```python
from build123d import *

# Parameters (mm, degrees)
F0_R          = 2
F1_DEPTH      = 20
F3_DEPTH      = 3
F3_DEPTH_BACK = 3
F6_DEPTH      = 1
F9_DEPTH      = 1
F10_DEPTH     = 20


with BuildPart() as f1:
    # F0 (on Front) → F1 (new body)
    with BuildSketch(Plane.XZ):
        with BuildLine():
            ThreePointArc((-3, 0), (0, -3), (3, 0))
            ThreePointArc((3, 0), (2.1213203436, 2.1213203436), (0, 3))
            ThreePointArc((0, 3), (-2.1213203436, 2.1213203436), (-3, 0))
        make_face()
        Circle(F0_R, mode=Mode.SUBTRACT)
    extrude(amount=F1_DEPTH)

    # F2 (on Right) → F3 (join, two sides)
    with BuildSketch(Plane.YZ) as f3_sk:
        Polygon((-5.2886751346, -7.6961524227), (-2, -2), (-3.1547005384, -2), (-6.1547005384, -7.1961524227), align=None)
        Polygon((-9.1547005384, -7.1961524227), (-6.1547005384, -2), (-7.3094010768, -2), (-10.0207259422, -6.6961524227), align=None)
    extrude(amount=F3_DEPTH)
    extrude(f3_sk.sketch, amount=-F3_DEPTH_BACK)

    # F5 (on offset) → F6 (join)
    with BuildSketch(Plane(origin=(0, -0.6339745962, 0.3660254038), x_dir=(-1, 0, 0), z_dir=(0, 0.8660254038, -0.5))):
        Polygon((3, -4), (3, 0), (1.5, -4), align=None)
        Polygon((-1.5, -4), (-3, 0), (-3, -4), align=None)
    extrude(amount=-F6_DEPTH)

    # F8 (on offset) → F9 (join)
    with BuildSketch(Plane(origin=(0, -3.75, 2.1650635095), x_dir=(-1, 0, 0), z_dir=(0, 0.8660254038, -0.5))):
        Polygon((3, -6), (3, -2.5), (1.5, -6), align=None)
        Polygon((-3, -6), (-1.5, -6), (-3, -2.5), align=None)
    extrude(amount=-F9_DEPTH)

    # F0 (on Front) → F10 (join)
    with BuildSketch(Plane.XZ):
        with BuildLine():
            ThreePointArc((-3, 0), (0, -3), (3, 0))
            ThreePointArc((3, 0), (2.1213203436, 2.1213203436), (0, 3))
            ThreePointArc((0, 3), (-2.1213203436, 2.1213203436), (-3, 0))
        make_face()
        Circle(F0_R, mode=Mode.SUBTRACT)
        with BuildLine():
            ThreePointArc((0, 3), (2.1213203436, 2.1213203436), (3, 0))
            Line((3, 0), (3, 3))
            Line((3, 3), (0, 3))
        make_face()
        with BuildLine():
            ThreePointArc((-3, 0), (-2.1213203436, 2.1213203436), (0, 3))
            Line((0, 3), (-3, 3))
            Line((-3, 3), (-3, 0))
        make_face()
    extrude(amount=F10_DEPTH)


solid = f1.part
```
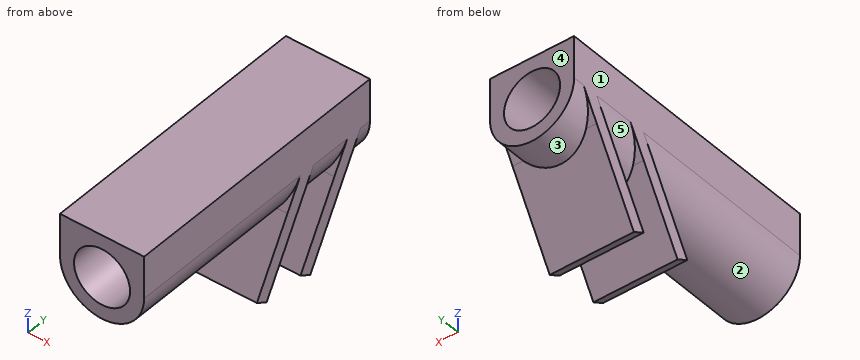
Check sheet for the modelled part. Datum: model origin and axes. Units: mm. Face numbers are marked on the shaded views. A direction names the side the tool comes from. Give positions to 0.01 mm unless a question says otherwise; leave off trailing zeros. Loops run counter-clockwise (first coordinate to the right, second up) from the corner with the lowest first, then second, coordinate; pieces in that order, holes last. Notation, with made-up numbers: (-6, 68.5) - (10, 68.5) arc R14 ccw to (10, 87.5) - close; hole circle Ø2 at (81.25, 82). An arc over 180 degrees is marked (long way). One line per question, with ' | ' between items. Start each with the question number.
1. Cross-section at A-A, the plane x = -0.5. Enter the section's corners in (y, z), plus the area to 3 significant figures.
2. Cross-section at B-B, the plane z = -5.75. Enter the section's corners in (x, y), plus the area to 3 significant figures.
3. Set-up check for the marked faces 4 and 5: record each of +Z, -Z, +X, -X, +Y, -Y from which the full face is reachable in a straight line by a thin tool's end or side.
4. Draft check along Z on the marked faces 1, 2 and 3. Enter one of: released by +Z, released by -Z, zero draft, split by the parting line, or undercut.
5. Cross-section at D-D, the plane x = 0.75. Enter the section's corners in (y, z).
6. Cross-section at C-C, the plane y = -17.25. Enter the section's corners in (x, z).
7. Gauge pin test, flat ends, axial feed: pin 1 Ø1 at (x, z) = (2, -4.5) entering from +Y; pin 2 Ø1.5 at (x, z) = (2, -2.5) entering from +Y. Record the tip position at first contact, or that the pin passes through.
8. Material ranges on line 1 along Z through (x, y) = (-1.5, -9); line 2 along Z through (x, y) = (0, -11); line 3 along Z through (x, y) = (-0.5, -4.25), recorded low to high. Write a range as [from, to].
Check result:
1) outline: (-20, -2.96) - (-7.86, -2.96) - (-10.02, -6.7) - (-9.15, -7.2) - (-6.71, -2.96) - (-3.71, -2.96) - (-6.15, -7.2) - (-5.29, -7.7) - (-2.55, -2.96) - (0, -2.96) - (0, -1.94) - (-20, -1.94) - close; (-20, 1.94) - (0, 1.94) - (0, 3) - (-20, 3) - close | area: 51.5 mm2
2) outline: (-3, -9.47) - (3, -9.47) - (3, -8.32) - (-3, -8.32) - close; (-3, -5.32) - (3, -5.32) - (3, -4.17) - (-3, -4.17) - close | area: 13.9 mm2
3) face 4: +Z, -Z, +X, -X, +Y | face 5: none
4) face 1: zero draft | face 2: undercut | face 3: released by -Z
5) outline: (-20, -2.9) - (-7.83, -2.9) - (-10.02, -6.7) - (-9.15, -7.2) - (-6.68, -2.9) - (-3.68, -2.9) - (-6.15, -7.2) - (-5.29, -7.7) - (-2.52, -2.9) - (0, -2.9) - (0, -1.85) - (-20, -1.85) - close; (-20, 1.85) - (0, 1.85) - (0, 3) - (-20, 3) - close
6) outline: (-3, 0) arc R3 ccw to (3, 0) - (3, 3) - (-3, 3) - close; hole circle Ø4 at (0, 0)
7) pin 1: stops at y = -3.15 | pin 2: stops at y = 0
8) line 1: z = [-6.93, -4.93], [-2.6, -1.32], [1.32, 3] | line 2: z = [-3, -2], [2, 3] | line 3: z = [-5.9, -3.9], [-2.96, -1.94], [1.94, 3]
